from build123d import *

# Parameters (mm, degrees)
CYLINDER010_R     = 1.25
CYLINDER010_DEPTH = 20
CYLINDER011_R     = 1.25
CYLINDER011_DEPTH = 20
BOX009_W          = 13
BOX009_H          = 6.8
BOX009_DEPTH      = 6
FILLET002_R       = 2
CYLINDER004_R     = 1.25
CYLINDER004_DEPTH = 7
CYLINDER002_R     = 1.25
CYLINDER002_DEPTH = 7
CYLINDER003_R     = 1.25
CYLINDER003_DEPTH = 7
CYLINDER_R        = 1.25
CYLINDER_DEPTH    = 7
BOX002_W          = 190
BOX002_H          = 68
BOX002_DEPTH      = 3
CYLINDER005_R     = 4
CYLINDER005_DEPTH = 6.3
CYLINDER006_R     = 4
CYLINDER006_DEPTH = 6.3
CYLINDER001_R     = 4
CYLINDER001_DEPTH = 6.3
BOX_W             = 216
BOX_H             = 80
BOX_DEPTH         = 3
CYLINDER007_R     = 4
CYLINDER007_DEPTH = 6.3
BOX003_W          = 2
BOX003_H          = 68
BOX003_DEPTH      = 2
BOX004_W          = 190
BOX004_H          = 2
BOX004_DEPTH      = 2
BOX021_W          = 13
BOX021_H          = 6.8
BOX021_DEPTH      = 6
FILLET002004_R    = 2


with BuildPart() as cylinder009:
    # Cylinder010 → Cylinder010 (new body)
    with BuildSketch(Plane(origin=(0, 30.5, 4), x_dir=(0, 0, -1), z_dir=(1, 0, 0))):
        Circle(CYLINDER010_R)
    extrude(amount=CYLINDER010_DEPTH)


with BuildPart() as fusion005:
    # Cylinder011 → Cylinder011 (new body)
    with BuildSketch(Plane(origin=(204, 30.5, 4), x_dir=(0, 0, -1), z_dir=(1, 0, 0))):
        Circle(CYLINDER011_R)
    extrude(amount=CYLINDER011_DEPTH)

    # Fusion005: union Cylinder009
    add(cylinder009.part)


with BuildPart() as fillet002:
    # Box009 → Box009 (new body)
    with BuildSketch(Plane(origin=(2, 29, 0), x_dir=(1, 0, 0), z_dir=(0, 0, 1))):
        with Locations((6.5, 3.4)):
            Rectangle(BOX009_W, BOX009_H)
    extrude(amount=BOX009_DEPTH)

    # Fillet002
    fillet002_edges = [fillet002.edges().sort_by_distance(p)[0] for p in [
        (8.5, 29, 6),
        (8.5, 35.8, 6),
    ]]
    fillet(fillet002_edges, radius=FILLET002_R)


with BuildPart() as fillet002_1:
    # Fillet002 placement: moved
    add(fillet002.part.moved(Location((0, -2, 0))))


with BuildPart() as screwhole003:
    # Cylinder004 → Cylinder004 (new body)
    with BuildSketch(Plane(origin=(214, 9.5, 0), x_dir=(1, 0, 0), z_dir=(0, 0, 1))):
        Circle(CYLINDER004_R)
    extrude(amount=CYLINDER004_DEPTH)


with BuildPart() as screwhole001:
    # Cylinder002 → Cylinder002 (new body)
    with BuildSketch(Plane(origin=(6, 71.2, 0), x_dir=(1, 0, 0), z_dir=(0, 0, 1))):
        Circle(CYLINDER002_R)
    extrude(amount=CYLINDER002_DEPTH)


with BuildPart() as screwhole002:
    # Cylinder003 → Cylinder003 (new body)
    with BuildSketch(Plane(origin=(214, 71.2, 0), x_dir=(1, 0, 0), z_dir=(0, 0, 1))):
        Circle(CYLINDER003_R)
    extrude(amount=CYLINDER003_DEPTH)


with BuildPart() as screwhole:
    # Cylinder → Cylinder (new body)
    with BuildSketch(Plane(origin=(6, 9.5, 0), x_dir=(1, 0, 0), z_dir=(0, 0, 1))):
        Circle(CYLINDER_R)
    extrude(amount=CYLINDER_DEPTH)


with BuildPart() as baseholes:
    # Box002 → Box002 (new body)
    with BuildSketch(Plane(origin=(15, 6, 1), x_dir=(1, 0, 0), z_dir=(0, 0, 1))):
        with Locations((95, 34)):
            Rectangle(BOX002_W, BOX002_H)
    extrude(amount=BOX002_DEPTH)

    # Fusion: union ScrewHole003, ScrewHole001, ScrewHole002, ScrewHole
    add(screwhole003.part)
    add(screwhole001.part)
    add(screwhole002.part)
    add(screwhole.part)


with BuildPart() as cylinder005:
    # Cylinder005 → Cylinder005 (new body)
    with BuildSketch(Plane(origin=(6, 71.2, 0), x_dir=(1, 0, 0), z_dir=(0, 0, 1))):
        Circle(CYLINDER005_R)
    extrude(amount=CYLINDER005_DEPTH)


with BuildPart() as cylinder006:
    # Cylinder006 → Cylinder006 (new body)
    with BuildSketch(Plane(origin=(214, 71.2, 0), x_dir=(1, 0, 0), z_dir=(0, 0, 1))):
        Circle(CYLINDER006_R)
    extrude(amount=CYLINDER006_DEPTH)


with BuildPart() as cylinder001:
    # Cylinder001 → Cylinder001 (new body)
    with BuildSketch(Plane(origin=(6, 9.5, 0), x_dir=(1, 0, 0), z_dir=(0, 0, 1))):
        Circle(CYLINDER001_R)
    extrude(amount=CYLINDER001_DEPTH)


with BuildPart() as base:
    # Box → Box (new body)
    with BuildSketch(Plane(origin=(2, 0, 0), x_dir=(1, 0, 0), z_dir=(0, 0, 1))):
        with Locations((108, 40)):
            Rectangle(BOX_W, BOX_H)
    extrude(amount=BOX_DEPTH)


with BuildPart() as basesubstraction:
    # Cylinder007 → Cylinder007 (new body)
    with BuildSketch(Plane(origin=(214, 9.5, 0), x_dir=(1, 0, 0), z_dir=(0, 0, 1))):
        Circle(CYLINDER007_R)
    extrude(amount=CYLINDER007_DEPTH)

    # Fusion001: union Cylinder005, Cylinder006, Cylinder001, Base
    add(cylinder005.part)
    add(cylinder006.part)
    add(cylinder001.part)
    add(base.part)

    # Cut: cut BaseHoles
    add(baseholes.part, mode=Mode.SUBTRACT)


with BuildPart() as reinforce:
    # Box003 → Box003 (new body)
    with BuildSketch(Plane(origin=(111, 6, 1), x_dir=(1, 0, 0), z_dir=(0, 0, 1))):
        with Locations((1, 34)):
            Rectangle(BOX003_W, BOX003_H)
    extrude(amount=BOX003_DEPTH)


with BuildPart() as reinforce001:
    # Box004 → Box004 (new body)
    with BuildSketch(Plane(origin=(15, 39, 1), x_dir=(1, 0, 0), z_dir=(0, 0, 1))):
        with Locations((95, 1)):
            Rectangle(BOX004_W, BOX004_H)
    extrude(amount=BOX004_DEPTH)


with BuildPart() as bottom:
    # Box021 → Box021 (new body)
    with BuildSketch(Plane(origin=(2, 29, 0), x_dir=(1, 0, 0), z_dir=(0, 0, 1))):
        with Locations((6.5, 3.4)):
            Rectangle(BOX021_W, BOX021_H)
    extrude(amount=BOX021_DEPTH)

    # Fillet002004
    fillet002004_edges = [bottom.edges().sort_by_distance(p)[0] for p in [
        (8.5, 29, 6),
        (8.5, 35.8, 6),
    ]]
    fillet(fillet002004_edges, radius=FILLET002004_R)


with BuildPart() as bottom_1:
    # Fillet002004 placement: moved
    add(bottom.part.moved(Location((203, -2, 0))))

    # Fusion008: union Fillet002, BaseSubstraction, Reinforce, Reinforce001
    add(fillet002_1.part)
    add(basesubstraction.part)
    add(reinforce.part)
    add(reinforce001.part)

    # Cut001006: cut Fusion005
    add(fusion005.part, mode=Mode.SUBTRACT)


solid = bottom_1.part
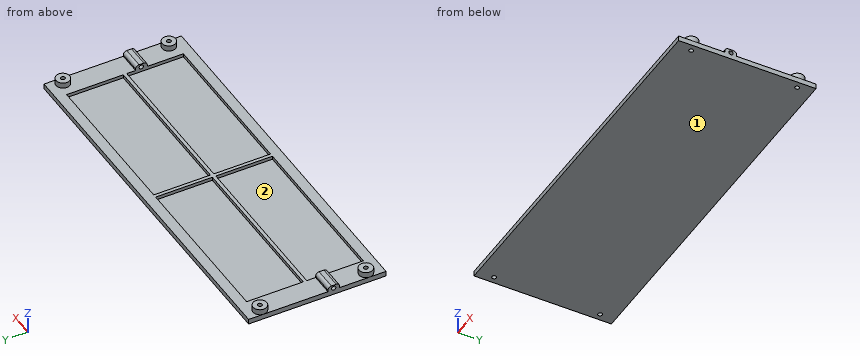
Check sheet for the modelled part. Datum: model origin and axes. Units: mm. Face numbers are marked on the shaded views. Coordinates: 2 decimals unless noted, no trailing zeros. Loops run counter-clockwise (first coordinate to the right, second up) from the corner with the lowest first, then second, coordinate; pieces in that order, holes last. Notation, with made-up numbers: (-9.5, -13) -> (0.5, -13) arc R17 cw to (0.5, 3) -> close; hole circle Ø1 at (25.25, 84). An arc over 180 degrees is marked (long way). Write item = value, one per line. Start each with the question number.
1. Section check A-A on y = 63. Record the cut outline in (x, z), then the cut area to 3 significant figures.
2. Draft check along X on the marked faces 1 and 2. Enter one of: released by +X, released by -X, zero draft, split by the parting line, or undercut.
3. Material ranges on line 1 (X direction, y = 9.5, z = 5); line 2 (X direction, y = 11, z = 1.75); line 3 (X direction, y = 71.2, z = 1.5), recorded low to high.
4. Section check B-B on x = 191.5. Record the cut outline in (y, z), then the cut area to 3 significant figures.
5. Depth check by flat-ended pin: P1, Ø2.5, axis at y = 21.5, z = 4, coming from the -X side; P2, Ø24, axis at x = 85.5, y = 43.5, coming from the +Z side; P3, Ø0.8, axis at x = 210.5, z = 3.5, coming from the -Y side; P4, Ø12, axis at x = 126, y = 66.5, coming from the +Z side. Enter the tip coordinate at first touch or a pass-through.
Responses:
q1.outline = (2, 0) -> (218, 0) -> (218, 3) -> (205, 3) -> (205, 1) -> (113, 1) -> (113, 3) -> (111, 3) -> (111, 1) -> (15, 1) -> (15, 3) -> (2, 3) -> close
q1.area = 272 mm2
q2.face_1 = zero draft
q2.face_2 = undercut
q3.line_1 = 2 to 4.75, 7.25 to 10, 210 to 212.75, 215.25 to 218
q3.line_2 = 2 to 15, 111 to 113, 205 to 218
q3.line_3 = 2 to 4.75, 7.25 to 15, 111 to 113, 205 to 212.75, 215.25 to 218
q4.outline = (0, 0) -> (80, 0) -> (80, 3) -> (74, 3) -> (74, 1) -> (41, 1) -> (41, 3) -> (39, 3) -> (39, 1) -> (6, 1) -> (6, 3) -> (0, 3) -> close
q4.area = 108 mm2
q5.P1 = 2
q5.P2 = 3
q5.P3 = 6.97
q5.P4 = 1
